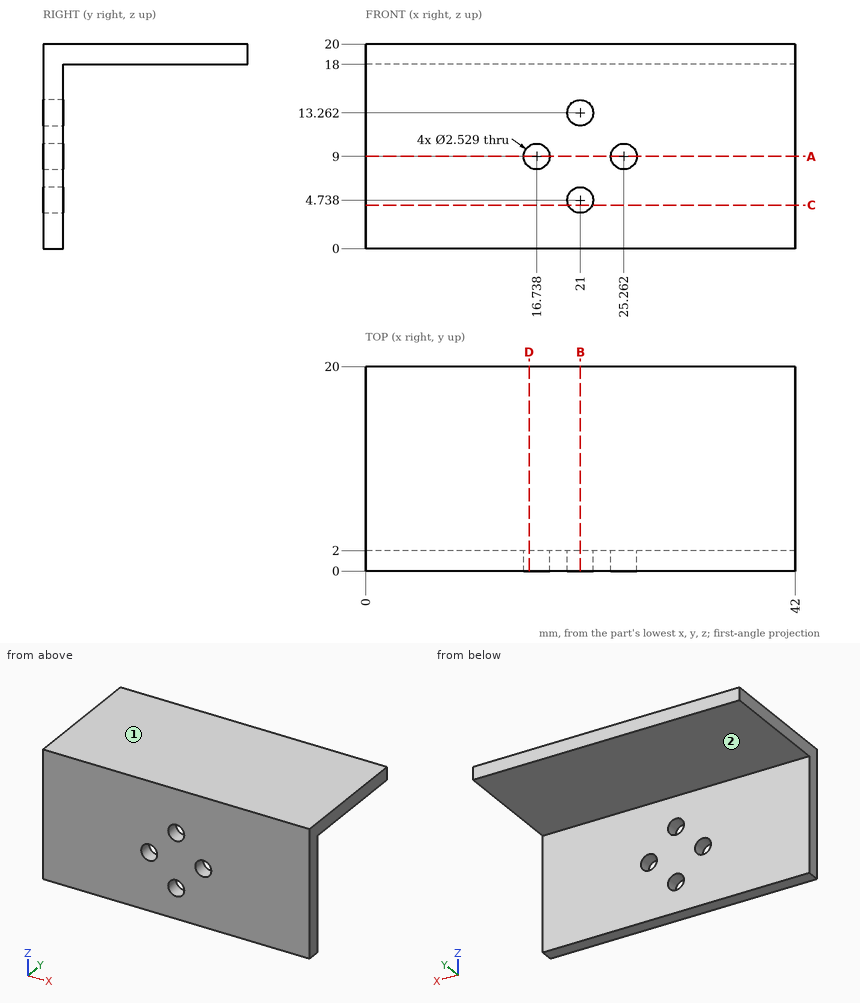
Geometry: see drawing. Coordinates: mm, zero at the bounding-box minimum. A direction names the side the tool comes from. Coordinates: 2 decimals unless noted, no trailing zeros. Loops run counter-clockwise (first coordinate to the right, second up) from the corner with the lowest first, then second, coordinate; pieces in that order, holes last. Notation, with made-up numbers: (18, 18) - (29, 18) arc R17 ccw to (29, 30) - close; hole circle Ø3 at (32.25, -18.5). An arc over 180 degrees is marked (long way). Put each result on its own line as item: value. Start each with the question number.
Q1. Cut plane D-D, the plane x = 16. Return loops of the section in (y, z), and give its area (3 significant figures).
Q2. Cut plane C-C, the plane z = 4.25. Return loops of the section in (x, y).
Q3. Line query: line 1 (X direction, y = 1.25, z = 9); line 2 (Z direction, x = 36, y = 14.75); line 3 (Y direction, x = 22, z = 11.75). Output: solid intervals per line, ascending.
Q4. Cut plane B-B, the plane x = 21. Return loops of the section in (y, z), and give its area (3 significant figures).
Q5. Set-up query: the marked faces 1 and 2. Return all of +Z, -Z, +X, -X, +Y, -Y with unobstructed straight access to the full face (end or side cutting, diameter ignored); none if empty.
Q6. Pin query (flat end, axial travel): pin 1 Ø4 at (x, z) = (27, 5) entering from +Y; pin 2 Ø3 at (x, z) = (16.5, 15.5) entering from -Y; pin 3 Ø2 at (y, z) = (10, 16) entering from -X. Return the tip coordinate at first contact, or that it passes through.
Q7. Cut plane A-A, the plane z = 9. Return loops of the section in (x, y).
Filled sheet:
1. outline: (0, 0) - (2, 0) - (2, 7.97) - (0, 7.97) - close; (0, 10.03) - (2, 10.03) - (2, 18) - (20, 18) - (20, 20) - (0, 20) - close
1. area: 71.9 mm²
2. outline: (0, 0) - (19.83, 0) - (19.83, 2) - (0, 2) - close; (22.17, 0) - (42, 0) - (42, 2) - (22.17, 2) - close
3. line 1: 0 to 15.47, 18 to 24, 26.53 to 42
3. line 2: 18 to 20
3. line 3: 0 to 2
4. outline: (0, 0) - (2, 0) - (2, 3.47) - (0, 3.47) - close; (0, 6) - (2, 6) - (2, 12) - (0, 12) - close; (0, 14.53) - (2, 14.53) - (2, 18) - (20, 18) - (20, 20) - (0, 20) - close
4. area: 65.9 mm²
5. face 1: +Z, +X, -X, +Y, -Y
5. face 2: -Z, +X, -X, +Y
6. pin 1: y = 2
6. pin 2: y = 0
6. pin 3: through
7. outline: (0, 0) - (15.47, 0) - (15.47, 2) - (0, 2) - close; (18, 0) - (24, 0) - (24, 2) - (18, 2) - close; (26.53, 0) - (42, 0) - (42, 2) - (26.53, 2) - close
